Verification items for the finished model (mm, model axes). Face numbers are marked on the shaded views. A direction names the side the tool comes from. Coordinates: 2 decimals unless noted, no trailing zeros. Order: outer loops, then holes, each group sorted by start corner. A loop starts at its lowest first (then second) coordinate and runs counter-clockwise, first axis right, second up. Notation, with made-up numbers: M 43,84 L 91,84 A38 cw 91,123 Z; hole C 57.5,36.5 d1. An arc over 180 degrees is marked long. Return JSON: item names as keys, results as strings. Group by question number.
1. Section check C-C, the plane z = -10. Record the cut outline in (x, y) (3 decimals).
2. Section check B-B, the plane x = -54.93. Record the cut outline in (y, z) (3 decimals).
3. Section check D-D, the plane y = 57.21. Give the number of separate pieces and of enclosed holes in the cut face, plus the area to 3 significant figures.
4. Mould release check, pull along Y, two halves, no side actions. Record for the marked faces 5, 6 and 7: +Y half, -Y half, draft (parallel to the pull), parting line (faces both ways), or undercut.
5. Section check A-A, the plane x = -19. Record the cut outline in (y, z).
6. Set-up check for the marked faces 1, 2, 3 and 4: record each of +Z, -Z, +X, -X, +Y, -Y from which the full face is reachable in a straight line by a thin tool's end or side.
7. Material ranges on line 1 along Y through (x, z) = (-38.93, 13.05); line 2 along X through (y, z) = (64, -8) (3 decimals); line 3 along Z through (x, y) = (-43.5, 57) (3 decimals), recorded low to high.
8. Gauge pin test, flat ends, axial feed: pin 1 (2 mm diameter, centred on x = -19.5, y = 35, fed in from +Z); pin 2 (1.6 mm diameter, centred on x = 3, y = 33.5, fed in from -Z); pin 3 (12 mm diameter, centred on x = -29.5, y = 55, fed in from +Z) (3 decimals); pin 4 (16.5 mm diameter, centred on x = -49, z = 3.5, fed in from -Y). Record the tip position at first contact, or that the pin passes through.
```python
from build123d import *

# Parameters (mm, degrees)
SKETCH_1_R           = 3.05
SKETCH_1_R_2         = 1.05
EXTRUDE_1_DEPTH      = 3.5
SKETCH_2_W           = 16
SKETCH_2_H           = 36
EXTRUDE_2_DEPTH      = 3.5
SKETCH_4_W           = 16
SKETCH_4_H           = 36
EXTRUDE_3_DEPTH      = 41.43
CUT_EXTRUDE_1_DEPTH  = 2
SKETCH_6_W           = 23
SKETCH_6_H           = 16
EXTRUDE_4_DEPTH      = 19.21
EXTRUDE_7_DEPTH      = 12.5
EXTRUDE_7_DEPTH_BACK = 10
SKETCH_9_W           = 3.515
SKETCH_9_H           = 10
EXTRUDE_8_DEPTH      = 20
EXTRUDE_9_DEPTH      = 3
SKETCH_11_R          = 1.05
CUT_EXTRUDE_2_DEPTH  = 31.5
SKETCH_12_W          = 15
SKETCH_12_H          = 6.433017237
CUT_EXTRUDE_3_DEPTH  = 94.183551258
CUT_EXTRUDE_4_REACH  = 76.726
SKETCH_13_W          = 11.984921516
SKETCH_13_H          = 8
SKETCH_14_W          = 13.03
SKETCH_14_H          = 7.5
CUT_EXTRUDE_5_DEPTH  = 98.004196945
CUT_EXTRUDE_6_REACH  = 84.547
SKETCH_15_W          = 6
SKETCH_15_H          = 15
SKETCH_17_W          = 20
SKETCH_17_H          = 12.5
CUT_EXTRUDE_11_DEPTH = 11.625
CUT_EXTRUDE_12_DEPTH = 10.125
FILLET_2_R           = 1
FILLET_3_R           = 1
FILLET_5_R           = 1
FILLET_7_R           = 1


with BuildPart() as part:
    # Sketch 1 → Extrude 1 (new body)
    with BuildSketch(Plane(origin=(0, 0, 0), x_dir=(1, 0, 0), z_dir=(0, 1, 0))):
        with BuildLine():
            Line((0, 8), (-15, 8))
            Line((-15, 8), (-15, -8))
            Line((-15, -8), (0, -8))
            ThreePointArc((0, -8), (8, 0), (0, 8))
        make_face()
        with Locations(Location((0, 0, 0), (0, 0, 270))):
            Circle(SKETCH_1_R, mode=Mode.SUBTRACT)
        with Locations(Location((-4.242640687, 4.242640687, 0), (0, 0, 270))):
            Circle(SKETCH_1_R_2, mode=Mode.SUBTRACT)
        with Locations(Location((-4.242640687, -4.242640687, 0), (0, 0, 270))):
            Circle(SKETCH_1_R_2, mode=Mode.SUBTRACT)
        with Locations(Location((4.242640687, -4.242640687, 0), (0, 0, 90))):
            Circle(SKETCH_1_R_2, mode=Mode.SUBTRACT)
        with Locations(Location((4.242640687, 4.242640687, 0), (0, 0, 90))):
            Circle(SKETCH_1_R_2, mode=Mode.SUBTRACT)
    extrude(amount=EXTRUDE_1_DEPTH)


with BuildPart() as body_2:
    # Mirror 4: mirrored copy
    add(part.part.mirror(Plane.ZX.offset(18)))


with BuildPart() as part_1:
    add(part.part)

    add(body_2.part)  # Extrude 2 merges body 2
    # Sketch 2 → Extrude 2 (add)
    with BuildSketch(Plane.ZY.offset(15)):
        with Locations((0, 18)):
            Rectangle(SKETCH_2_W, SKETCH_2_H)
    extrude(amount=EXTRUDE_2_DEPTH)

    # Sketch 4 → Extrude 3 (add)
    with BuildSketch(Plane.ZY.offset(18.5)):
        with Locations((0, 18)):
            Rectangle(SKETCH_4_W, SKETCH_4_H)
    extrude(amount=EXTRUDE_3_DEPTH)

    # Sketch 5 → Cut-Extrude 1 (cut)
    with BuildSketch(Plane.XZ.offset(-32.5)):
        with BuildLine():
            Line((0, 3.05), (8.87097286, 3.05))
            Line((8.87097286, 3.05), (10.441846702, -3.05))
            Line((10.441846702, -3.05), (0, -3.05))
            ThreePointArc((0, -3.05), (3.05, 0), (0, 3.05))
        make_face()
    extrude(amount=-CUT_EXTRUDE_1_DEPTH, mode=Mode.SUBTRACT)

    # Sketch 6 → Extrude 4 (add)
    with BuildSketch(Plane(origin=(0, 36, 0), x_dir=(1, 0, 0), z_dir=(0, 1, 0))):
        with Locations((-48.43, 0)):
            Rectangle(SKETCH_6_W, SKETCH_6_H)
    extrude(amount=EXTRUDE_4_DEPTH)

    # Sketch 8 → Extrude 7 (add, two sides: drawn at the far end of the back side and taken through both)
    with BuildSketch(Plane(origin=(0, 55.21, 0), x_dir=(1, 0, 0), z_dir=(0, 1, 0)).offset(-EXTRUDE_7_DEPTH_BACK)):
        Polygon((-56.93, 11.515), (-36.93, 11.515), (-36.93, 14.515), (-59.93, 14.515), (-59.93, 11.515), (-59.93, 0), (-59.93, -11.515), (-59.93, -14.515), (-36.93, -14.515), (-36.93, -11.515), (-56.93, -11.515), (-56.93, -8), (-56.93, 8), align=None)
    extrude(amount=EXTRUDE_7_DEPTH + EXTRUDE_7_DEPTH_BACK)

    # Sketch 9 → Extrude 8 (add)
    with BuildSketch(Plane(origin=(-56.93, 0, 0), x_dir=(0, 0, -1), z_dir=(1, 0, 0))):
        with Locations((-9.7575, 50.21)):
            Rectangle(SKETCH_9_W, SKETCH_9_H)
        with Locations((9.7575, 50.21)):
            Rectangle(SKETCH_9_W, SKETCH_9_H)
    extrude(amount=EXTRUDE_8_DEPTH)

    # Sketch 10 → Extrude 9 (add)
    with BuildSketch(Plane(origin=(-36.93, 0, 0), x_dir=(0, 0, -1), z_dir=(1, 0, 0))):
        Polygon((-11.515, 67.71), (11.515, 67.71), (14.515, 67.71), (14.515, 45.21), (8, 45.21), (-8, 45.21), (-14.515, 45.21), (-14.515, 67.71), align=None)
    extrude(amount=EXTRUDE_9_DEPTH)

    # Sketch 11 → Cut-Extrude 2 (cut, symmetric)
    with BuildSketch(Plane(origin=(0, 0, 11.515), x_dir=(-1, 0, 0), z_dir=(0, 0, -1))):
        with Locations((38.93, 57.21)):
            Circle(SKETCH_11_R)
        with Locations((54.93, 57.21)):
            Circle(SKETCH_11_R)
    extrude(amount=CUT_EXTRUDE_2_DEPTH, both=True, mode=Mode.SUBTRACT)

    # Sketch 12 → Cut-Extrude 3 (cut, through all)
    with BuildSketch(Plane(origin=(0, 0, -8), x_dir=(-1, 0, 0), z_dir=(0, 0, -1))):
        with BuildLine():
            Line((22, 30.5), (22, 5.5))
            ThreePointArc((22, 5.5), (41.52562419, 12.569250972), (52, 30.5))
            Line((52, 30.5), (22, 30.5))
        make_face()
        with Locations((48.43, 38.993491382)):
            Rectangle(SKETCH_12_W, SKETCH_12_H)
        with BuildLine():
            Line((59.918359247, 35.060355361), (67.982296312, -21.171088437))
            Line((67.982296312, -21.171088437), (30.309681235, -1.008567897))
            ThreePointArc((30.309681235, -1.008567897), (51.317225959, 11.93373394), (59.918359247, 35.060355361))
        make_face()
    extrude(amount=-CUT_EXTRUDE_3_DEPTH, mode=Mode.SUBTRACT)

    # Sketch 13 → Cut-Extrude 4 (cut, up to next)
    with BuildSketch(Plane.XZ.offset(-42.21), mode=Mode.PRIVATE) as cut_extrude_4_sk1:
        with Locations((-46.937539242, 0)):
            Rectangle(SKETCH_13_W, SKETCH_13_H)
    cut_extrude_4_tool1 = extrude(cut_extrude_4_sk1.sketch, amount=-CUT_EXTRUDE_4_REACH, mode=Mode.PRIVATE) & part_1.part
    add(cut_extrude_4_tool1.solids().sort_by_distance((-46.937539, 42.21, 0))[0], mode=Mode.SUBTRACT)

    # Sketch 14 → Cut-Extrude 5 (cut, through all)
    with BuildSketch(Plane.ZY.offset(59.93)):
        with Locations((0, 58.96)):
            Rectangle(SKETCH_14_W, SKETCH_14_H)
    extrude(amount=-CUT_EXTRUDE_5_DEPTH, mode=Mode.SUBTRACT)

    # Sketch 15 → Cut-Extrude 6 (cut, up to next)
    with BuildSketch(Plane(origin=(-15, 0, 0), x_dir=(0, 0, -1), z_dir=(1, 0, 0)), mode=Mode.PRIVATE) as cut_extrude_6_sk1:
        with Locations((0, 18)):
            Rectangle(SKETCH_15_W, SKETCH_15_H)
    cut_extrude_6_tool1 = extrude(cut_extrude_6_sk1.sketch, amount=-CUT_EXTRUDE_6_REACH, mode=Mode.PRIVATE) & part_1.part
    add(cut_extrude_6_tool1.solids().sort_by_distance((-15, 18, 0))[0], mode=Mode.SUBTRACT)

    # Sketch 17 → Cut-Extrude 11 (cut, symmetric)
    with BuildSketch(Plane(origin=(0, 0, 0), x_dir=(-1, 0, 0), z_dir=(0, 0, -1))):
        with Locations((46.93, 61.46)):
            Rectangle(SKETCH_17_W, SKETCH_17_H)
    extrude(amount=CUT_EXTRUDE_11_DEPTH, both=True, mode=Mode.SUBTRACT)

    # Sketch 18 → Cut-Extrude 12 (cut, symmetric)
    with BuildSketch(Plane.ZY.offset(46.93)):
        Polygon((-11.625, 55.21), (-6.515, 55.21), (-6.515, 62.71), (6.515, 62.71), (6.515, 55.21), (11.625, 55.21), (11.625, 67.71), (-11.625, 67.71), align=None)
    extrude(amount=CUT_EXTRUDE_12_DEPTH, both=True, mode=Mode.SUBTRACT)

    # Fillet 2
    fillet_2_edges = [part_1.edges().sort_by_distance(p)[0] for p in [
        (-46.93, 67.71, -11.625),
        (-46.93, 67.71, 11.625),
        (-36.805, 67.71, 0),
        (-57.055, 67.71, 0),
    ]]
    fillet(fillet_2_edges, radius=FILLET_2_R)

    # Fillet 3
    fillet_3_edges = [part_1.edges().sort_by_distance(p)[0] for p in [
        (-46.93, 67.71, -14.515),
        (-59.93, 67.71, 0),
        (-46.93, 67.71, 14.515),
        (-33.93, 67.71, 0),
    ]]
    fillet(fillet_3_edges, radius=FILLET_3_R)

    # Fillet 5
    # the kernel refuses this fillet: 1 mm, written as the material it takes off along each edge
    with BuildSketch(Plane(origin=(-58.93, 66.71, -13.515), x_dir=(-1, 0, 0), z_dir=(0, 0, -1))) as fillet_5_piece_1_section:
        Polygon((0, 0), (FILLET_5_R, 0), (FILLET_5_R, FILLET_5_R), (0, FILLET_5_R), align=None)
    fillet_5_piece_1 = extrude(amount=FILLET_5_R, mode=Mode.PRIVATE)
    fillet_5_piece_1 = fillet_5_piece_1 - Plane(origin=(-58.93, 66.71, -13.515), x_dir=(0.7071067811865475, -0.7071067811865475, 0), z_dir=(0, 0, -1)) * Sphere(FILLET_5_R, mode=Mode.PRIVATE)
    add(fillet_5_piece_1, mode=Mode.SUBTRACT)
    with BuildSketch(Plane(origin=(-34.93, 66.71, -13.515), x_dir=(1, 0, 0), z_dir=(0, 0, -1))) as fillet_5_piece_2_section:
        Polygon((0, 0), (FILLET_5_R, 0), (FILLET_5_R, -FILLET_5_R), (0, -FILLET_5_R), align=None)
    fillet_5_piece_2 = extrude(amount=FILLET_5_R, mode=Mode.PRIVATE)
    fillet_5_piece_2 = fillet_5_piece_2 - Plane(origin=(-34.93, 66.71, -13.515), x_dir=(-0.7071067811865475, -0.7071067811865475, 0), z_dir=(0, 0, -1)) * Sphere(FILLET_5_R, mode=Mode.PRIVATE)
    add(fillet_5_piece_2, mode=Mode.SUBTRACT)
    with BuildSketch(Plane(origin=(-58.93, 66.71, 13.515), x_dir=(0, 0, 1), z_dir=(-1, 0, 0))) as fillet_5_piece_3_section:
        Polygon((0, 0), (FILLET_5_R, 0), (FILLET_5_R, FILLET_5_R), (0, FILLET_5_R), align=None)
    fillet_5_piece_3 = extrude(amount=FILLET_5_R, mode=Mode.PRIVATE)
    fillet_5_piece_3 = fillet_5_piece_3 - Plane(origin=(-58.93, 66.71, 13.515), x_dir=(0, -0.7071067811865475, -0.7071067811865475), z_dir=(-1, 0, 0)) * Sphere(FILLET_5_R, mode=Mode.PRIVATE)
    add(fillet_5_piece_3, mode=Mode.SUBTRACT)
    with BuildSketch(Plane(origin=(-34.93, 66.71, 13.515), x_dir=(0, 0, 1), z_dir=(1, 0, 0))) as fillet_5_piece_4_section:
        Polygon((0, 0), (FILLET_5_R, 0), (FILLET_5_R, -FILLET_5_R), (0, -FILLET_5_R), align=None)
    fillet_5_piece_4 = extrude(amount=FILLET_5_R, mode=Mode.PRIVATE)
    fillet_5_piece_4 = fillet_5_piece_4 - Plane(origin=(-34.93, 66.71, 13.515), x_dir=(0, -0.7071067811865475, -0.7071067811865475), z_dir=(1, 0, 0)) * Sphere(FILLET_5_R, mode=Mode.PRIVATE)
    add(fillet_5_piece_4, mode=Mode.SUBTRACT)
    with BuildSketch(Plane(origin=(-59.93, 42.71, 14.515), x_dir=(0, 0, -1), z_dir=(0, 1, 0)), Plane(origin=(-59.93, 42.71, -14.515), x_dir=(1, 0, 0), z_dir=(0, 1, 0)), Plane(origin=(-33.93, 66.71, -14.515), x_dir=(-1, 0, 0), z_dir=(0, -1, 0))) as fillet_5_piece_5:
        with BuildLine():
            CenterArc((FILLET_5_R, -FILLET_5_R), FILLET_5_R, 90, 90)
            Line((0, -FILLET_5_R), (0, 0))
            Line((0, 0), (FILLET_5_R, 0))
        make_face()
    extrude(amount=24, mode=Mode.SUBTRACT)
    with BuildSketch(Plane(origin=(-33.93, 42.71, 14.515), x_dir=(0, 0, -1), z_dir=(0, 1, 0))) as fillet_5_piece_6:
        with BuildLine():
            CenterArc((FILLET_5_R, FILLET_5_R), FILLET_5_R, 180, 90)
            Line((0, FILLET_5_R), (0, 0))
            Line((0, 0), (FILLET_5_R, 0))
        make_face()
    extrude(amount=24, mode=Mode.SUBTRACT)

    # Fillet 7
    fillet_7_edges = [part_1.edges().sort_by_distance(p)[0] for p in [
        (-22, 18, 8),
        (-41.52562419, 12.569250972, 8),
        (-37, 30.5, 8),
        (-37, 30.5, -8),
        (-22, 18, -8),
        (-41.52562419, 12.569250972, -8),
    ]]
    fillet(fillet_7_edges, radius=FILLET_7_R)


solid = part_1.part
```
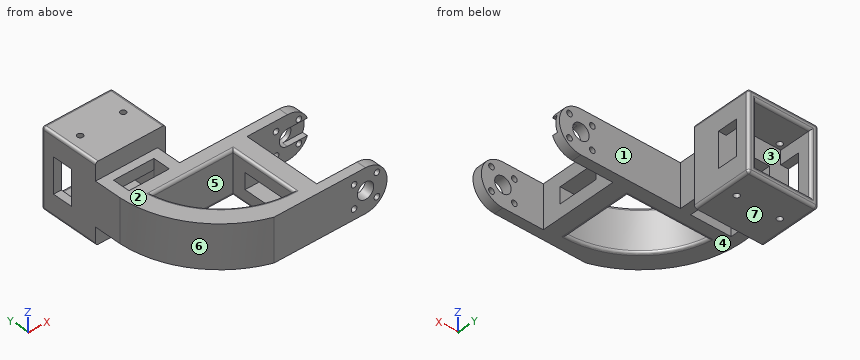
Answers follow:
{
 "1": {"outline": "M -59.93,45.21 L -33.93,45.21 L -33.93,66.71 A1 ccw -34.93,67.71 L -35.805,67.71 A1 ccw -36.805,66.71 L -36.805,55.21 L -57.055,55.21 L -57.055,66.71 A1 ccw -58.055,67.71 L -58.93,67.71 A1 ccw -59.93,66.71 Z"},
 "2": {"outline": "M 17.177,-8 L 35.777,-8 L 35.777,8 L 17.177,8 Z; M 42.21,-8 L 45.21,-8 L 45.21,-14.515 L 56.16,-14.515 L 56.16,-11.625 L 55.21,-11.625 L 55.21,11.625 L 56.16,11.625 L 56.16,14.515 L 45.21,14.515 L 45.21,8 L 42.21,8 Z; M 58.26,-14.515 L 66.71,-14.515 A1 ccw 67.71,-13.515 L 67.71,-12.625 A1 ccw 66.71,-11.625 L 58.26,-11.625 Z; M 58.26,11.625 L 66.71,11.625 A1 ccw 67.71,12.625 L 67.71,13.515 A1 ccw 66.71,14.515 L 58.26,14.515 Z"},
 "3": {"separate pieces": "6", "enclosed holes": "0", "area": "184 mm^2"},
 "4": {"face 5": "undercut", "face 6": "-Y half", "face 7": "draft"},
 "5": {"outline": "M 0,-8 L 36,-8 L 36,8 L 0,8 Z; hole M 10.5,-3 L 25.5,-3 L 25.5,3 L 10.5,3 Z"},
 "6": {"face 1": "+Z, -Z, +X", "face 2": "+Z, +X, -X, -Y", "face 3": "none", "face 4": "-Z, +X, -X, -Y"},
 "7": {"line 1": "45.21 to 56.16, 58.26 to 67.71", "line 2": "-59.93 to -57.055, -36.805 to -33.93", "line 3": "-14.515 to -11.625, 11.625 to 14.515"},
 "8": {"pin 1": "z = 8", "pin 2": "z = -7.69", "pin 3": "z = 14.515", "pin 4": "y = 3.03"}
}
